from build123d import *

# Parameters (mm, degrees)
BOSS_EXTRUDE1_DEPTH = 10.16
BOSS_EXTRUDE2_DEPTH = 10.16
CHAMFER1_SIZE       = 2.54


with BuildPart() as part:
    # Sketch3 → Boss-Extrude1 (new body)
    with BuildSketch(Plane(origin=(0, 0, 0), x_dir=(0, 0, -1), z_dir=(1, 0, 0))):
        Polygon((-101.845577666, -9.102652747), (-95.495577666, -9.102652747), (-95.495577666, 9.947347253), (-89.145577666, 9.947347253), (-89.145577666, 22.647347253), (-51.045577666, 22.647347253), (-51.045577666, 9.947347253), (-44.695577666, 9.947347253), (-44.695577666, -9.102652747), (-38.345577666, -9.102652747), (-38.345577666, 28.997347253), (-101.845577666, 28.997347253), align=None)
    extrude(amount=BOSS_EXTRUDE1_DEPTH)

    # Sketch4 → Boss-Extrude2 (add)
    with BuildSketch(Plane(origin=(10.16, 0, 0), x_dir=(0, 0, -1), z_dir=(1, 0, 0))):
        with BuildLine():
            Line((-101.845577666, -4.906246043), (-101.845577666, 7.020940549))
            ThreePointArc((-101.845577666, 7.020940549), (-93.844577666, 1.057347253), (-101.845577666, -4.906246043))
        make_face()
        with BuildLine():
            Line((-38.345577666, -4.906246043), (-38.345577666, 7.020940549))
            ThreePointArc((-38.345577666, 7.020940549), (-46.346577666, 1.057347253), (-38.345577666, -4.906246043))
        make_face()
    extrude(amount=-BOSS_EXTRUDE2_DEPTH)

    # Chamfer1
    chamfer1_edges = [part.edges().sort_by_distance(p)[0] for p in [
        (5.08, 9.947347253, 44.695577666),
        (5.08, 9.947347253, 95.495577666),
    ]]
    chamfer(chamfer1_edges, length=CHAMFER1_SIZE)


solid = part.part
CAD build for the part. Positions are in the model's coordinates, mm. A direction names the side the tool comes from. Round coordinates to 2 decimals unless told otherwise and drop trailing zeros. Write each loop counter-clockwise with the first axis right and the second up, starting at its lowest first coordinate (ties: lowest second). Pieces come first, ordered by that corner, then holes. Notation, with made-up numbers: (53, -34.75) -> (95, -34.75) arc R11 ccw to (95, -14.75) -> close; hole circle Ø9 at (-31.75, 81). An arc over 180 degrees is marked (long way). Answer as a JSON object with one key per item and string values.
(1) Probe probe 1 along Z at (x, y) = (9.25, 11); probe 2 along Y at (x, z) = (6.75, 82); probe 3 along Z at (x, y) = (5, 5.5). List the from-to ranges inside material, lowest first. Write a range as [from, to].
Reported:
{"probe 1": "z = [38.35, 51.05], [89.15, 101.85]", "probe 2": "y = [22.65, 29]", "probe 3": "z = [38.35, 44.7], [95.5, 101.85]"}
(2) Which spindle directions (+Z, -Z, +X, -X, +Y, -Y) get a long thin tool onto all of the face, cutting with end or side? Do faces 4 (the face through (0, 23, 71)), 5 (the face through (5.009, 8.66, 94.243)), 6 (the face through (5, 22.647, 70)). Say none if no direction does.
Reported:
{"face 4": "+Z, -Z, -X, +Y, -Y", "face 5": "+X, -X", "face 6": "+X, -X, -Y"}
(3) Band-saw the part on C-C, the plane z = 45.5. List the corners of the cut face in (x, y).
Reported:
{"outline": "(0, -2.08) -> (10.16, -2.08) -> (10.16, 4.19) -> (0, 4.19) -> close; (0, 8.21) -> (10.16, 8.21) -> (10.16, 29) -> (0, 29) -> close"}
(4) Band-saw the part on A-A, the plane y = 16.5. List the corners of the cut face in (x, z), then the cut area to 3 significant figures.
Reported:
{"outline": "(0, 38.35) -> (10.16, 38.35) -> (10.16, 51.05) -> (0, 51.05) -> close; (0, 89.15) -> (10.16, 89.15) -> (10.16, 101.85) -> (0, 101.85) -> close", "area": "258 mm^2"}
(5) Band-saw the part on D-D, the plane z = 91. List the corners of the cut face in (x, y).
Reported:
{"outline": "(0, 9.95) -> (10.16, 9.95) -> (10.16, 29) -> (0, 29) -> close"}
(6) Band-saw the part on B-B, the plane x = 5. List the corners of the cut face in (y, z), then the cut area to 3 significant figures.
Reported:
{"outline": "(-9.1, 38.35) -> (29, 38.35) -> (29, 101.85) -> (-9.1, 101.85) -> (-9.1, 95.5) -> (-3.16, 95.5) arc R6.22 ccw to (5.28, 95.5) -> (7.41, 95.5) -> (9.95, 92.96) -> (9.95, 89.15) -> (22.65, 89.15) -> (22.65, 51.05) -> (9.95, 51.05) -> (9.95, 47.24) -> (7.41, 44.7) -> (5.28, 44.7) arc R6.22 ccw to (-3.16, 44.7) -> (-9.1, 44.7) -> close", "area": "993 mm^2"}
(7) Two-plate mould, pull along Z, no slides. Class faces 1 (the face through (5, 10, 38.346)), 2 (the face through (5, -6, 95.496)), 3 (the face through (5, 28.997, 70)): +Z half, -Z half, draft (parallel to the pull), parting line (faces both ways), or undercut.
Reported:
{"face 1": "-Z half", "face 2": "undercut", "face 3": "draft"}
(8) Pin check, flat tips, straight feed: P1, Ø5, axis at x = 6.5, z = 65, coming from the -Y side; P2, Ø8, axis at y = 14.5, z = 88, coming from the +X side; P3, Ø4, axis at x = 3.5, z = 91.5, coming from the -Y side; P4, Ø4, axis at x = 3.5, z = 49.5, coming from the -Y side. Stop position of each tip, or through.
Reported:
{"P1": "stops at y = 22.65", "P2": "stops at x = 10.16", "P3": "stops at y = 9.4", "P4": "stops at y = 9.95"}
